Geometry check sheet. Reference: the model listing, model coordinates, mm. A direction names the side the tool comes from. Coordinates: 2 decimals unless noted, no trailing zeros. Order: outer loops, then holes, each group sorted by start corner. A loop starts at its lowest first (then second) coordinate and runs counter-clockwise, first axis right, second up.
```python
from build123d import *

# Parameters (mm, degrees)
F1_DEPTH = 970
F2_W     = 35
F2_H     = 30
F3_DEPTH = 2.3
F4_W     = 2.4
F4_H     = 1
F5_DEPTH = 30.001
F7_DEPTH = 970


with BuildPart() as f1:
    # F0 (on Right) → F1 (new body)
    with BuildSketch(Plane.YZ):
        Polygon((0, 20), (0, 0), (2.3, 0), (2.3, 17.7), (27.7, 17.7), (27.7, 0), (30, 0), (30, 20), align=None)
    extrude(amount=F1_DEPTH)

    # F2 (on face) → F3 (cut)
    with BuildSketch(Plane.XY.offset(20)):
        with Locations((17.5, 15)):
            Rectangle(F2_W, F2_H)
        with Locations((952.5, 15)):
            Rectangle(F2_W, F2_H)
    extrude(amount=-F3_DEPTH, mode=Mode.SUBTRACT)

    # F4 (on face) → F5 (cut, through all)
    with BuildSketch(Plane.XZ):
        with Locations((33.8, 0.5)):
            Rectangle(F4_W, F4_H)
        with Locations((6.2, 0.5)):
            Rectangle(F4_W, F4_H)
        with Locations((936.2, 0.5)):
            Rectangle(F4_W, F4_H)
        with Locations((963.8, 0.5)):
            Rectangle(F4_W, F4_H)
    extrude(amount=-F5_DEPTH, mode=Mode.SUBTRACT)


with BuildPart() as f7:
    # F6 (on Right) → F7 (new body)
    with BuildSketch(Plane.YZ):
        Polygon((-5, 20), (95, 20), (174.204771, 10.246291), (176.204771, 10), (257.409543, 0), (273.650497, 0), (95, 22), (-5, 22), align=None)
        Polygon((176.204771, 10), (174.204771, 10.246291), (174.204771, 0), (176.204771, 0), align=None)
    extrude(amount=F7_DEPTH)


solid = f7.part
```
Item 1: Sectioned sample at C-C (y = 231.5). Record the cut outline in (x, z).
Item 2: Depth check by flat-ended pin: P1, Ø11.5, axis at x = 555, z = 4, coming from the -Y side; P2, Ø8, axis at x = 349, y = 189, coming from the -Z side; P3, Ø1.5, axis at x = 759, y = 25, coming from the -Z side. Enter the tip coordinate at first touch or a pass-through.
Item 3: Sectioned sample at B-B (x = 342.5). Record the cut outline in (y, z).
Item 4: Release check for a two-part mould opening along Y. For faces 3 (the face through (478.21, 216.24, 5.07)), 4 (the face through (478, 265, 0)), 5 (the face through (478.21, 185.576, 10.846)), 6 (the face through (478.21, 134.05, 15.19)) record: pulls with the +Y half, pulls with the -Y half, needs draft (parallel to the pull), parting line crosses it, or undercut.
Item 5: Thickness scan on line 1 along Z through (x, y) = (171, 67); line 2 along Z through (x, y) = (248.5, 117). Record the ranges inside material, lowest first.
Item 6: Tool access check on faces 1 (the face through (478, 44, 20)), 2 (the face through (478, 46, 22)). Record the directions out of +Z, -Z, +X, -X, +Y, -Y that give a thin tool (end or side, any length) a straight path to the whole face; none if there is none.
Item 7: Sectioned sample at A-A (z = 5.75). Record the cut outline in (x, y).
Geometry check:
1. outline: (0, 3.19) - (970, 3.19) - (970, 5.19) - (0, 5.19) - close
2. P1: stops at y = 174.2
2. P2: stops at z = 7.93
2. P3: stops at z = 20
3. outline: (-5, 20) - (95, 20) - (174.2, 10.25) - (174.2, 0) - (176.2, 0) - (176.2, 10) - (257.41, 0) - (273.65, 0) - (95, 22) - (-5, 22) - close
4. face 3: undercut
4. face 4: needs draft
4. face 5: pulls with the +Y half
4. face 6: pulls with the -Y half
5. line 1: z = 20 to 22
5. line 2: z = 17.29 to 19.29
6. face 1: -Z, +X, -X, -Y
6. face 2: +Z, +X, -X, +Y, -Y
7. outline: (0, 174.2) - (970, 174.2) - (970, 176.2) - (0, 176.2) - close; (0, 210.72) - (970, 210.72) - (970, 226.96) - (0, 226.96) - close
